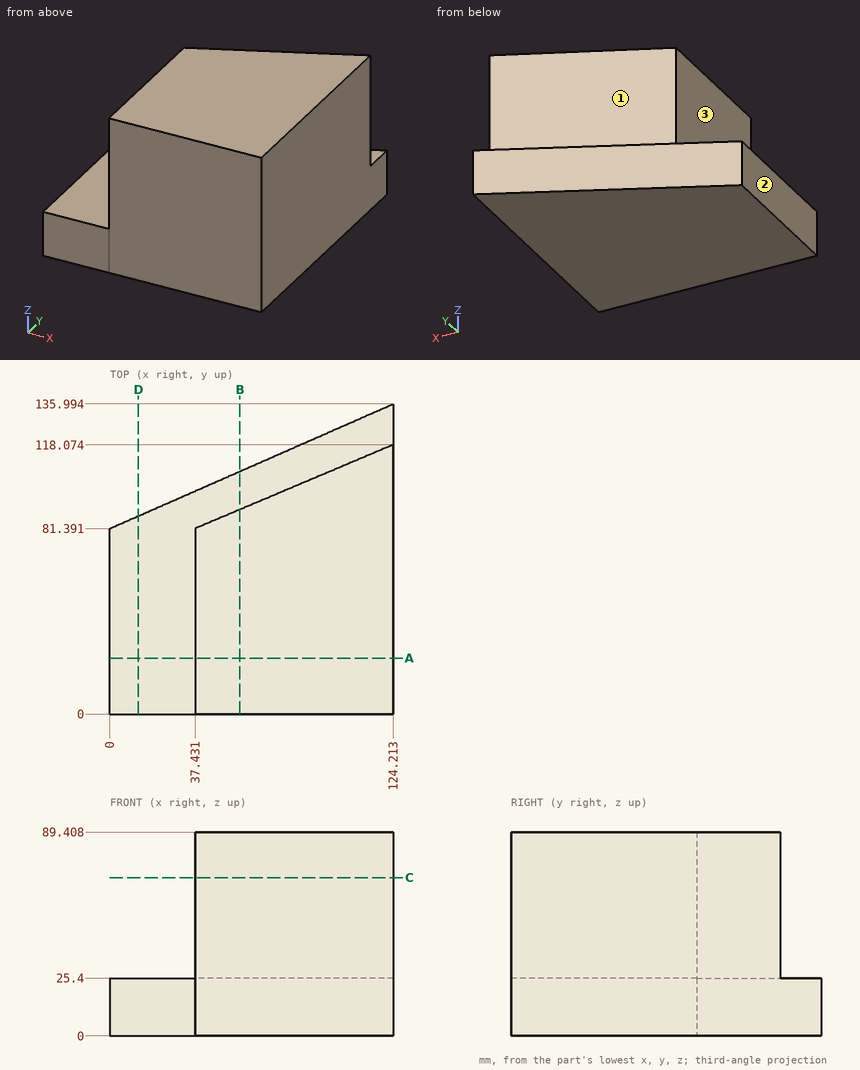
The drawing under review shows one solid part. Ordinate dimensions are in mm from its lowest x, y, z. A direction names the side the tool comes from. Round coordinates to 2 decimals unless told otherwise and drop trailing zeros. Loops run counter-clockwise (first coordinate to the right, second up) from the corner with the lowest first, then second, coordinate; pieces in that order, holes last. Notation, with made-up numbers: (63.5, 41) - (82.5, 41) arc R25 cw to (82.5, 69) - close; hole circle Ø1 at (-7.5, 19). An arc over 180 degrees is marked (long way). One line per question, with ' | ' between items.
1. Clearance check with flat-ended pins moving along their axes: P1, Ø4, axis at y = 120.5, z = 67.5, coming from the +X side; P2, Ø2, axis at y = 85.5, z = 71.5, coming from the -X side (1 decimal); P3, Ø4, axis at x = 54, z = 64.5, coming from the +Y side. State where each tip first meets the part, or that it passes through.
Results are:
P1: passes through | P2: stops at x = 44.8 | P3: stops at y = 89.24
2. For L1, parallel to X at y = 55.5, z = 65.5; L2, parallel to Z at x = 94.5, y = 118; L3, parallel to Y at x = 65.5, z = 82 (1 decimal), list the stretches that pass through material, from the lowest coordinate up. Write a range as [from, to].
Results are:
L1: x = [37.43, 124.21] | L2: z = [0, 25.4] | L3: y = [0, 93.3]
3. For the marked faces 1, 2 and 3, list the 3-axis set-ups (+Z, -Z, +X, -X, +Y, -Y) from which the entire face can be reached by the end or side of a thin tool; tool diameter is ignored.
Results are:
face 1: +Z, -X, +Y | face 2: +Z, -Z, -X, +Y, -Y | face 3: +Z, -X, +Y, -Y
4. We need section D-D, the plane x = 12.5. State the section outline as (y, z) points, and give its area (3 significant figures).
Results are:
outline: (0, 0) - (86.89, 0) - (86.89, 25.4) - (0, 25.4) - close | area: 2,210 mm²
5. We need section C-C, the plane z = 69.5. State the section outline as (x, y) points.
Results are:
outline: (37.43, 0) - (124.21, 0) - (124.21, 118.07) - (37.43, 81.39) - close
6. We need section B-B, the plane x = 57. State the section outline as (y, z) points, and give its area (3 significant figures).
Results are:
outline: (0, 0) - (106.45, 0) - (106.45, 25.4) - (89.66, 25.4) - (89.66, 89.41) - (0, 89.41) - close | area: 8,440 mm²
7. We need section A-A, the plane y = 24.5. State the section outline as (x, z) points, and give its area (3 significant figures).
Results are:
outline: (0, 0) - (124.21, 0) - (124.21, 89.41) - (37.43, 89.41) - (37.43, 25.4) - (0, 25.4) - close | area: 8,710 mm²
